For this review, take the finished solid that the model builds, in its own axes (mm). Give positions to 0.01 mm unless a question says otherwise; leave off trailing zeros. Order: outer loops, then holes, each group sorted by start corner. A loop starts at its lowest first (then second) coordinate and runs counter-clockwise, first axis right, second up. Notation, with made-up numbers: M -10,81.5 L 49,81.5 A17 cw 49,99.5 Z; hole C 41,75 d10. An arc over 180 degrees is marked long. Use CSV: the item, a comma, the result in double quotes. Start each with the question number.
(1) Consider section B-B (x = 17.5). Write out the cut boundary in (y, z), and give its area (3 significant figures).
(2) Consider section A-A (z = -31.5). Write out the cut boundary in (x, y).
(3) Clearance check with flat-ended pins moving along their axes: P1, Ø2.5, axis at x = 62, z = -37, coming from the +Y side; P2, Ø1.8, axis at x = 0, z = 37, coming from the -Y side; P3, Ø3, axis at x = -62, z = -37, coming from the -Y side; P4, Ø0.9, axis at x = 15.5, y = -1.5, coming from the -Z side. State where each tip first meets the part, or that it passes through.
(4) Wall thickness on L1, parallel to Z at x = -62, y = 0.9; L2, parallel to Z at x = 0, y = 0.6; L3, parallel to X at y = -1.55, z = 20: over which ranges is each line inside the solid? List them lowest first. Write a range as from..to.
(5) Consider section C-C (y = -1.25). Write out the cut boundary in (x, z), and give its area (3 significant figures).
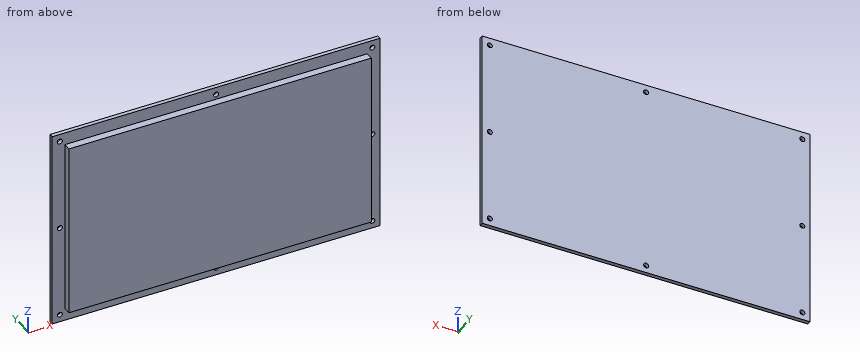
```python
from build123d import *

# Parameters (mm, degrees)
F0_W     = 120
F0_H     = 70
F2_DEPTH = 3
F1_W     = 130
F1_H     = 80
F3_DEPTH = 1.6
F4_D     = 2


with BuildPart() as f2:
    # F0 (on Front) → F2 (new body)
    with BuildSketch(Plane.XZ):
        Rectangle(F0_W, F0_H)
    extrude(amount=F2_DEPTH)

    # F1 (on Front) → F3 (join)
    with BuildSketch(Plane.XZ):
        Rectangle(F1_W, F1_H)
    extrude(amount=-F3_DEPTH)

    # F4 (through all)
    with Locations(Plane.XZ):
        with Locations((62, 37), (62, 0), (62, -37), (0, -37), (0, 37), (-62, 37), (-62, 0), (-62, -37)):
            Hole(F4_D / 2)


solid = f2.part
```
Check result:
1,outline,"M -3,-35 L 0,-35 L 0,-40 L 1.6,-40 L 1.6,40 L 0,40 L 0,35 L -3,35 Z"
1,area,"338 mm^2"
2,outline,"M -65,0 L -60,0 L -60,-3 L 60,-3 L 60,0 L 65,0 L 65,1.6 L -65,1.6 Z"
3,P1,"stops at y = 1.6"
3,P2,"passes through"
3,P3,"stops at y = 0"
3,P4,"stops at z = -35"
4,L1,"z = -40..-38, -36..-1, 1..36, 38..40"
4,L2,"z = -40..-38, -36..36, 38..40"
4,L3,"x = -60..60"
5,outline,"M -60,-35 L 60,-35 L 60,35 L -60,35 Z"
5,area,"8,400 mm^2"
